Geometry: final body of the model. Coordinates: model frame, mm. Face numbers are marked on the shaded views. Give positions to 0.01 mm unless a question says otherwise; leave off trailing zeros. Loops run counter-clockwise (first coordinate to the right, second up) from the corner with the lowest first, then second, coordinate; pieces in that order, holes last. Notation, with made-up numbers: M 18,23 L 36,23 A30 cw 36,61 Z; hole C 9,-8.75 d9. An arc over 180 degrees is marked long. One line per question, with ' | ' between items. Start each with the question number.
from build123d import *

# Parameters (mm, degrees)
EXTRUDE_1_DEPTH     = 6
CUT_EXTRUDE_START   = -6
CUT_EXTRUDE_1_DEPTH = 1
CUT_EXTRUDE_3_DEPTH = 3
SKETCH_5_OUTSIDE_W  = 281.366
SKETCH_5_OUTSIDE_H  = 83.498
CUT_EXTRUDE_2_DEPTH = 124.858535656
HOLE_WIZARD_M4_1_D  = 4.3
FILLET_3_R          = 2


with BuildPart() as part:
    # ｽｹｯﾁ1 → ﾎﾞｽ - 押し出し1 (new body)
    with BuildSketch(Plane.XY):
        with BuildLine():
            Line((-74.445215618, -8), (-65.183849372, -8))
            ThreePointArc((-65.183849372, -8), (-59.472431605, -21.788582233), (-45.683849372, -27.5))
            Line((-45.683849372, -27.5), (45.683849372, -27.5))
            ThreePointArc((45.683849372, -27.5), (59.472431605, -21.788582233), (65.183849372, -8))
            Line((65.183849372, -8), (74.445215618, -8))
            ThreePointArc((74.445215618, -8), (83.886790831, -21.023796042), (99.183849372, -26))
            Line((99.183849372, -26), (116.183849372, -26))
            Line((116.183849372, -26), (116.183849372, -34))
            Line((116.183849372, -34), (66.183849372, -42.5))
            Line((66.183849372, -42.5), (-66.183849372, -42.5))
            Line((-66.183849372, -42.5), (-116.183849372, -34))
            Line((-116.183849372, -34), (-116.183849372, -26))
            Line((-116.183849372, -26), (-99.183849372, -26))
            ThreePointArc((-99.183849372, -26), (-83.886790831, -21.023796042), (-74.445215618, -8))
        make_face()
    extrude(amount=-EXTRUDE_1_DEPTH)

    # ｽｹｯﾁ1<5> → ｶｯﾄ - 押し出し1 (cut)
    with BuildSketch(Plane.XY.offset(CUT_EXTRUDE_START)):
        with BuildLine():
            Line((-66.183849372, -8), (-72.183849372, -8))
            Line((-72.183849372, -8), (-72.183849372, -27))
            Line((-72.183849372, -27), (-116.183849372, -27))
            Line((-116.183849372, -27), (-116.183849372, -33))
            Line((-116.183849372, -33), (-72.183849372, -33))
            Line((-72.183849372, -33), (-72.183849372, -34))
            ThreePointArc((-72.183849372, -34), (-71.183849372, -35), (-70.183849372, -34))
            Line((-70.183849372, -34), (-68.183849372, -34))
            ThreePointArc((-68.183849372, -34), (-67.183849372, -35), (-66.183849372, -34))
            Line((-66.183849372, -34), (-66.183849372, -8))
        make_face()
        with BuildLine():
            Line((72.183849372, -8), (66.183849372, -8))
            Line((66.183849372, -8), (66.183849372, -34))
            ThreePointArc((66.183849372, -34), (67.183849372, -35), (68.183849372, -34))
            Line((68.183849372, -34), (70.183849372, -34))
            ThreePointArc((70.183849372, -34), (71.183849372, -35), (72.183849372, -34))
            Line((72.183849372, -34), (72.183849372, -33))
            Line((72.183849372, -33), (116.183849372, -33))
            Line((116.183849372, -33), (116.183849372, -27))
            Line((116.183849372, -27), (72.183849372, -27))
            Line((72.183849372, -27), (72.183849372, -8))
        make_face()
    extrude(amount=CUT_EXTRUDE_1_DEPTH, mode=Mode.SUBTRACT)

    # ｽｹｯﾁ1<6> → ｶｯﾄ - 押し出し3 (cut)
    with BuildSketch(Plane.XY.offset(CUT_EXTRUDE_START)):
        with BuildLine():
            Line((-58, -38.5), (-58, -42.5))
            Line((-58, -42.5), (-50, -42.5))
            Line((-50, -42.5), (-50, -38.5))
            ThreePointArc((-50, -38.5), (-54, -34.5), (-58, -38.5))
        make_face()
        with BuildLine():
            Line((-22, -38.5), (-22, -42.5))
            Line((-22, -42.5), (-14, -42.5))
            Line((-14, -42.5), (-14, -38.5))
            ThreePointArc((-14, -38.5), (-18, -34.5), (-22, -38.5))
        make_face()
        with BuildLine():
            Line((14, -38.5), (14, -42.5))
            Line((14, -42.5), (22, -42.5))
            Line((22, -42.5), (22, -38.5))
            ThreePointArc((22, -38.5), (18, -34.5), (14, -38.5))
        make_face()
        with BuildLine():
            Line((50, -38.5), (50, -42.5))
            Line((50, -42.5), (58, -42.5))
            Line((58, -42.5), (58, -38.5))
            ThreePointArc((58, -38.5), (54, -34.5), (50, -38.5))
        make_face()
    extrude(amount=CUT_EXTRUDE_3_DEPTH, mode=Mode.SUBTRACT)

    # ｽｹｯﾁ5 outside → ｶｯﾄ - 押し出し2 (cut, through all)
    with BuildSketch(Plane.XY):
        with Locations((0, -25.25)):
            Rectangle(SKETCH_5_OUTSIDE_W, SKETCH_5_OUTSIDE_H)
        with BuildLine():
            Line((-66.183849372, -27), (-61.183849372, -27))
            ThreePointArc((-61.183849372, -27), (-60.683849372, -27.5), (-60.183849372, -27))
            Line((-60.183849372, -27), (-60.183849372, -26))
            Line((-60.183849372, -26), (-55.183849372, -26))
            ThreePointArc((-55.183849372, -26), (-53.28004345, -30.596194078), (-48.683849372, -32.5))
            Line((-48.683849372, -32.5), (48.683849372, -32.5))
            ThreePointArc((48.683849372, -32.5), (53.28004345, -30.596194078), (55.183849372, -26))
            Line((55.183849372, -26), (60.183849372, -26))
            Line((60.183849372, -26), (60.183849372, -27))
            ThreePointArc((60.183849372, -27), (60.683849372, -27.5), (61.183849372, -27))
            Line((61.183849372, -27), (66.183849372, -27))
            Line((66.183849372, -27), (66.183849372, -42.5))
            Line((66.183849372, -42.5), (-66.183849372, -42.5))
            Line((-66.183849372, -42.5), (-66.183849372, -27))
        make_face(mode=Mode.SUBTRACT)
    extrude(amount=-CUT_EXTRUDE_2_DEPTH, mode=Mode.SUBTRACT)

    # M4 すきま穴1 (through all)
    with Locations(Plane(origin=(-54, -38.5, 0), x_dir=(1, 0, 0), z_dir=(0, 0, 1))):
        with Locations((0, 0), (36, 0), (72, 0), (108, 0)):
            Hole(HOLE_WIZARD_M4_1_D / 2)

    # ﾌｨﾚｯﾄ3
    fillet_3_edges = [part.edges().sort_by_distance(p)[0] for p in [
        (-58, -42.5, -4.5),
        (-50, -42.5, -4.5),
        (-22, -42.5, -4.5),
        (-14, -42.5, -4.5),
        (14, -42.5, -4.5),
        (22, -42.5, -4.5),
        (50, -42.5, -4.5),
        (58, -42.5, -4.5),
        (-66.183849372, -27, -3),
        (-55.183849372, -26, -3),
        (55.183849372, -26, -3),
        (66.183849372, -27, -3),
        (-66.183849372, -42.5, -3),
        (66.183849372, -42.5, -3),
    ]]
    fillet(fillet_3_edges, radius=FILLET_3_R)


solid = part.part
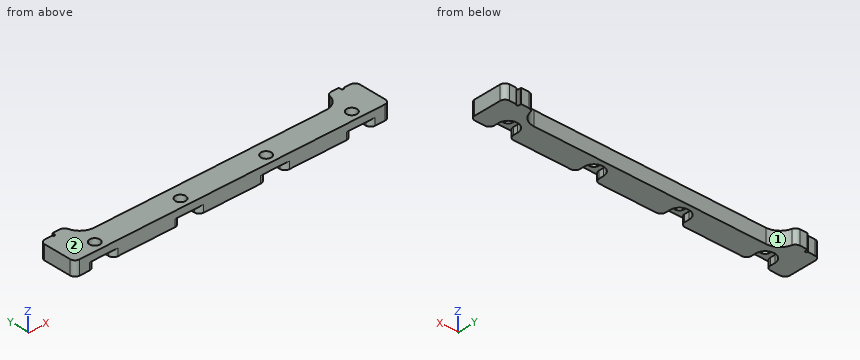
Q1. Section C-C, the plane x = -33.5. Output: boundary loops of the cut face in (y, z), plus the area to 3 significant figures.
Q2. Contact query for flat-ended pins moving along their axis: pin 1 (4 mm diameter, centred on x = -18, y = -40.5, fed in from -Z); pin 2 (2.5 mm diameter, centred on x = -62.5, z = -3.5, fed in from +Y); pin 3 (1.5 mm diameter, centred on y = -28, z = -4.5, fed in from -X). Output: stop coordinate, or through.
Q3. Section B-B, the plane z = -1.05. Output: boundary loops of the cut face in (x, y), plus the area to 3 significant figures.
Q4. Section A-A, the plane x = 18. Output: boundary loops of the cut face in (y, z).
Q5. Material intervals for L1, parallel to Y at x = 18, z = -0.65; L2, parallel to X at y = -36, z = -3.45; L3, parallel to X at y = -37.5, z = -3.3, sorted ascending.
Q6. Draft query along X for the marked faces 1 and 2. Return one class per face: released by +X, released by -X, zero draft, split by the parting line, or undercut.
Model answer:
1) outline: M -42.5,-6 L -32.5,-6 L -32.5,0 L -42.5,0 Z | area: 60.0 mm^2
2) pin 1: stops at z = -3 | pin 2: stops at y = -27 | pin 3: stops at x = -66.17
3) outline: M -66.18,-40.5 A2 ccw -64.18,-42.5 L 64.18,-42.5 A2 ccw 66.18,-40.5 L 66.18,-29 A2 ccw 64.18,-27 L 61.18,-27 A0.5 cw 60.18,-27 L 60.18,-26 L 56.95,-26 A2 ccw 55,-27.53 A6.5 cw 48.68,-32.5 L -48.68,-32.5 A6.5 cw -55,-27.53 A2 ccw -56.95,-26 L -60.18,-26 L -60.18,-27 A0.5 cw -61.18,-27 L -64.18,-27 A2 ccw -66.18,-29 Z; hole C -54,-38.5 d4.3; hole C -18,-38.5 d4.3; hole C 18,-38.5 d4.3; hole C 54,-38.5 d4.3 | area: 1,410 mm^2
4) outline: M -42.5,-3 L -40.65,-3 L -40.65,0 L -42.5,0 Z; M -36.35,-3 L -34.5,-3 L -34.5,-6 L -32.5,-6 L -32.5,0 L -36.35,0 Z
5) L1: y = -42.5 to -40.65, -36.35 to -32.5 | L2: x = -66.18 to -57.12, -50.88 to -21.12, -14.88 to 14.88, 21.12 to 50.88, 57.12 to 66.18 | L3: x = -66.18 to -57.87, -50.13 to -21.87, -14.13 to 14.13, 21.87 to 50.13, 57.87 to 66.18
6) face 1: undercut | face 2: zero draft
